Can you work these out from the model? Positions are in its coordinate system, mm. Face numbers are marked on the shaded views. A direction names the side the tool comes from. Round coordinates to 2 decimals unless told otherwise and drop trailing zeros. Loops run counter-clockwise (first coordinate to the right, second up) from the corner with the lowest first, then second, coordinate; pieces in that order, holes last. Notation, with made-up numbers: M -8.75,-32 L 1.25,-32 A4 ccw 1.25,-28 Z; hole C 86,66.25 d8. An arc over 180 degrees is marked long. Answer as CSV lines item,"result".
from build123d import *

# Parameters (mm, degrees)
F0_W      = 30
F0_H      = 27
F1_DEPTH  = 27
F2_SIZE   = 4
F4_D      = 5
F5_W      = 8
F5_H      = 23
F5_H_2    = 4
F6_DEPTH  = 2.1
F7_W      = 8
F7_H      = 28.8321655244
F7_H_2    = 23
F7_H_3    = 5.8321655244
F8_DEPTH  = 2.1
F9_W      = 8
F9_H      = 33.7052789075
F9_H_2    = 5.6568542495
F9_H_3    = 30.637866843
F10_DEPTH = 14.5
F12_D     = 4
F12_DEPTH = 4
F12_TIP   = 1.2017212381


with BuildPart() as f1:
    # F0 (on Front) → F1 (new body)
    with BuildSketch(Plane.XZ):
        Rectangle(F0_W, F0_H)
    extrude(amount=F1_DEPTH)

    # F2
    f2_edges = [f1.edges().sort_by_distance(p)[0] for p in [
        (0, 0, -13.5),
        (0, -27, 13.5),
    ]]
    chamfer(f2_edges, length=F2_SIZE)

    # F4 (through all)
    with Locations(Plane.XZ.offset(27)):
        with Locations((-10, -0.5), (10, -0.5)):
            Hole(F4_D / 2)

    # F5 (on face) → F6 (cut)
    with BuildSketch(Plane.XZ.offset(27)):
        with Locations((0, -2)):
            Rectangle(F5_W, F5_H)
        with Locations((0, 11.5)):
            Rectangle(F5_W, F5_H_2)
    extrude(amount=-F6_DEPTH, mode=Mode.SUBTRACT)

    # F7 (on face) → F8 (cut)
    with BuildSketch(Plane.XY.offset(13.5)):
        with Locations((0, 14.4160827622)):
            Rectangle(F7_W, F7_H)
        with Locations((0, -11.5)):
            Rectangle(F7_W, F7_H_2)
        with Locations((0, -25.9160827622)):
            Rectangle(F7_W, F7_H_3)
    extrude(amount=-F8_DEPTH, mode=Mode.SUBTRACT)

    # F9 (on face) → F10 (cut)
    with BuildSketch(Plane(origin=(0, 4.75, -4.75), x_dir=(-1, 0, 0), z_dir=(0, 0.7071067812, -0.7071067812))):
        with Locations((0, -29.2270081245)):
            Rectangle(F9_W, F9_H)
        with Locations((0, -9.545941546)):
            Rectangle(F9_W, F9_H_2)
        with Locations((0, 8.6014190002)):
            Rectangle(F9_W, F9_H_3)
    extrude(amount=-F10_DEPTH, mode=Mode.SUBTRACT)

    # F12
    with Locations(Plane.XZ.offset(24.9)):
        with Locations((0, -7.5), (0, 7.5)):
            Hole(F12_D / 2, depth=F12_DEPTH)
            with Locations((0, 0, -(F12_DEPTH + F12_TIP / 2))):  # 118° drill point
                Cone(0, F12_D / 2, F12_TIP, mode=Mode.SUBTRACT)


solid = f1.part
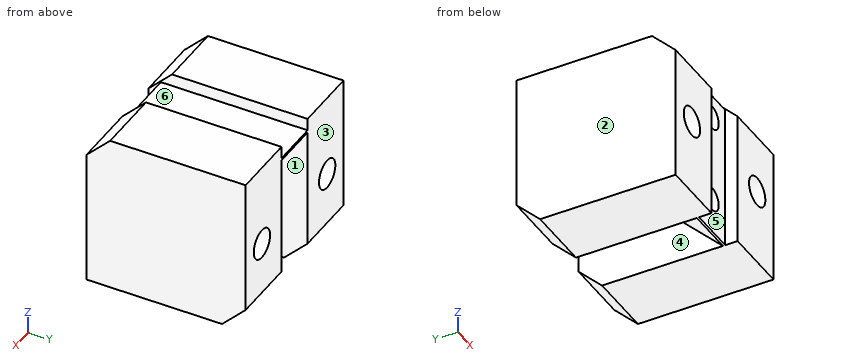
Item 1: We'd pull the mould along X, two halves only. Please class the marked faces 1, 2 and 3: released by +X, released by -X, zero draft, split by the parting line, or undercut.
Output:
face 1,"undercut"
face 2,"released by -X"
face 3,"zero draft"
Item 2: Will these pins go through, and if not, where does the flat tip stop? pin 1 (12 mm diameter, centred on x = 3.5, z = 2.5, fed in from -Y); pin 2 (2.5 mm diameter, centred on x = 0, z = -7.5, fed in from -Y); pin 3 (6.5 mm diameter, centred on x = 0, y = -15, fed in from +Z); pin 4 (4 mm diameter, centred on x = 0, z = 3, fed in from -Y).
Output:
pin 1,"stops at y = -27"
pin 2,"stops at y = -20.45"
pin 3,"stops at z = 11.4"
pin 4,"stops at y = -24.9"
Item 3: If we section it at B-B on y = -5: Write out the boundary of the cut face in (x, z).
Output:
outline,"M -15,-13.5 L -4,-13.5 L -4,6.01 L 4,6.01 L 4,-13.5 L 15,-13.5 L 15,13.5 L 4,13.5 L 4,11.4 L -4,11.4 L -4,13.5 L -15,13.5 Z; hole C -10,-0.5 d5; hole C 10,-0.5 d5"
Item 4: If we section it at C-C on z = -0.5: Write out the boundary of the cut face in (x, y), then the cut area to 3 significant figures.
Output:
outline,"M -15,-27 L -12.5,-27 L -12.5,0 L -15,0 Z; M -7.5,-27 L -4,-27 L -4,-24.9 L 4,-24.9 L 4,-27 L 7.5,-27 L 7.5,0 L 4,0 L 4,-11.51 L -4,-11.51 L -4,0 L -7.5,0 Z; M 12.5,-27 L 15,-27 L 15,0 L 12.5,0 Z"
area,"431 mm2"
Item 5: If we section it at D-D on x = 12: Write out the boundary of the cut face in (y, z).
Output:
outline,"M -27,-13.5 L -4,-13.5 L 0,-9.5 L 0,-2 L -27,-2 Z; M -27,1 L 0,1 L 0,13.5 L -23,13.5 L -27,9.5 Z"
Item 6: On a 3-axis mill with a long thin cutter (end or side, diameter ignored), from which of +Z, -Z, +X, -X, +Y, -Y can I reach the whole of each face in a straight line? I mean the marked faces 4, 5 and 6. Say none if no direction works.
Output:
face 4,"-Z, +Y"
face 5,"+Z, -Z, -Y"
face 6,"+Z, +Y, -Y"
Item 7: If I drill on line 1 along X through (y, z) = (-23.35, 7.5); line 2 along X through (y, z) = (-8.5, 11.5); line 3 along Z through (x, y) = (0, -23.15), over which ranges is the centre line in solid material (lowest first)? Write a range as from..to.
Output:
line 1,"x = -15..-2, 2..15"
line 2,"x = -15..-4, 4..15"
line 3,"z = -12.14..-9.5, -5.5..5.5, 9.5..11.4"
Item 8: If we section it at A-A on x = -10: Write out the boundary of the cut face in (y, z).
Output:
outline,"M -27,-13.5 L -4,-13.5 L 0,-9.5 L 0,-3 L -27,-3 Z; M -27,2 L 0,2 L 0,13.5 L -23,13.5 L -27,9.5 Z"
